CAD build for the part. Positions are in the model's coordinates, mm. Face numbers are marked on the shaded views. A direction names the side the tool comes from. Coordinates: 2 decimals unless noted, no trailing zeros. Loops run counter-clockwise (first coordinate to the right, second up) from the corner with the lowest first, then second, coordinate; pieces in that order, holes last. Notation, with made-up numbers: (-26, 24) - (20, 24) arc R13 cw to (20, 40) - close; hole circle Ø4 at (70.5, -7.5). An arc over 180 degrees is marked (long way). Put each result on its own line as item: value.
Autodesk Inventor part; units mm, degrees
ref_plane "YZ Plane" through (0, 0, 0) normal (1, 0, 0) x (0, 1, 0)
ref_plane "XZ Plane" through (0, 0, 0) normal (0, 1, 0) x (-1, 0, 0)
ref_plane "XY Plane" through (0, 0, 0) normal (0, 0, 1) x (1, 0, 0)
sketch "Sketch1" plane through (0, 0, 0) normal (0, 0, 1) x (1, 0, 0)
  line L0 (-490, 52) -> (490, 52)
  line L1 (490, 52) -> (490, 0)
  line L2 (490, 0) -> (-490, 0)
  line L3 (-490, 0) -> (-490, 52)
  point P0 (0, 0)
  point P1 (0, 0)
  dimension "d0" = 980
  dimension "d1" = 52
extrude "Plate1" add sketch "Sketch1" along normal blind 2
sketch "Sketch2" plane through (490, 2, 0) normal (0, -1, 0) x (1, 0, 0)
  line L0 (-980, 0) -> (0, 0)
  line L1 (0, 0) -> (0, 20)
  line L2 (0, 20) -> (-980, 20)
  line L3 (-980, 20) -> (-980, 0)
edge flange "Flange1" height 20 angle 90 thickness 2 bend radius 2.75 thickness toward (0, -1, 0) relief round relief width 2 relief depth 1 edges at (0, 0, 2) wall of the first edge with corners at (-490, 2, 0) (490, 2, 0) (490, 2, 20) (-490, 2, 20)
bend "Bend1"
corner "Corner1"
sketch "Sketch11" plane through (0, 0, 0) normal (0, 0, 1) x (1, 0, 0)
  line L0 (-490, 52) -> (490, 52)
  circle A0 centre (0, 52) radius 30
  line L1 (-490, 0) -> (490, 0)
  line L2 (246.05, 0) -> (243.95, 0)
  line L3 (243.95, 0) -> (243.95, 27)
  line L4 (243.95, 27) -> (246.05, 27)
  line L5 (246.05, 27) -> (246.05, 0)
  line L6 (-243.95, 0) -> (-246.05, 0)
  line L7 (-246.05, 0) -> (-246.05, 27) construction
  line L8 (-246.05, 27) -> (-243.95, 27) construction
  line L9 (-243.95, 27) -> (-243.95, 0) construction
  line L10 (0, 52) -> (0, 0)
  line L11 (246.05, 27) -> (246.05, 52)
  line L12 (243.95, 27) -> (243.95, 52)
  line L13 (-243.95, 27) -> (-243.95, 52) construction
  line L14 (-246.05, 27) -> (-246.05, 52) construction
  line L15 (-490, 0) -> (-490, 52)
  circle A1 centre (490, 52) radius 30
  line L16 (490, 52) -> (490, 0)
  point P0 (30, 52)
  point P1 (-30, 52)
  point P2 (-245, 27)
  point P3 (245, 27)
  point P4 (490, 22)
  point P5 (460, 52)
  point P6 (0, 22)
  dimension "d44" = 60
  dimension "d47" = 2.1
  dimension "d49" = 490
  dimension "d50" = 27
extrude "Extrusion4" cut sketch "Sketch11" along normal through all both and the other way through all contours L10 A0 L0 | A0 L10 L1 L15 L0 | L0 L11 L4 L12 picked at (-19.7493, 49.7748)
sketch "Sketch9" plane through (0, 0, 2) normal (0, 0, 1) x (1, 0, 0)
  line L0 (456.3279, 23.6801) -> (456.3279, 11.6801) construction
  line L1 (456.3279, 11.6801) -> (256.3279, 11.6801) construction
  line L2 (256.3279, 11.6801) -> (256.3279, 23.6801) construction
  line L3 (256.3279, 23.6801) -> (456.3279, 23.6801) construction
  line L4 (-490, 52) -> (490, 52)
  point P0 (0, 0)
  point P1 (1, 52)
  dimension "d38" = 200
  dimension "d39" = 12
mark "Mark3"
equation "\"d1\" = СПИНА_Стрингер_1_высота"
equation "\"d2\" = Thickness"
equation "\"d3\" = BendReliefWidth"
equation "\"d4\" = BendReliefDepth"
equation "\"d5\" = MinimumRemnant"
equation "\"d6\" = TransitionRadius"
equation "\"d9\" = BendRadius"
equation "\"d10\" = CornerReliefSize"
equation "\"d11\" = GapSize"
equation "\"d12\" = JacobiRadiusSize"
equation "\"BendReliefWidth\" = Thickness"
equation "\"BendReliefDepth\" = 0.5 * Thickness"
equation "\"CornerReliefSize\" = 4 * Thickness"
equation "\"MinimumRemnant\" = 2 * Thickness"
equation "\"TransitionRadius\" = BendRadius"
equation "\"JacobiRadiusSize\" = BendRadius"
equation "\"GapSize\" = Thickness"
properties part number "MSC 204 STRINGER BACK ^" material "Stainless Steel"
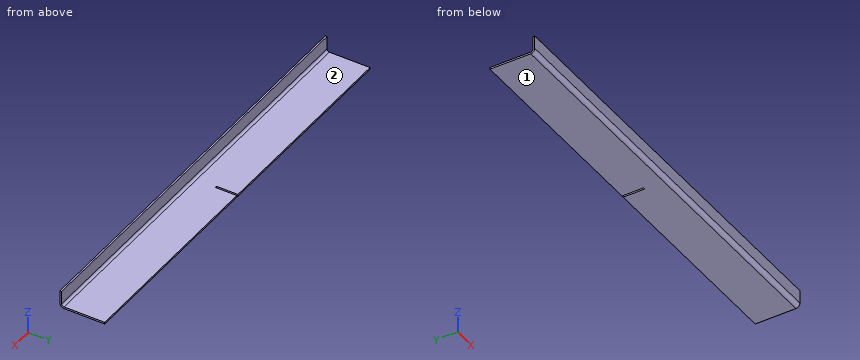
Q1. Slice it at A-A, the plane x = 141. Give the cut face in (y, z).
Determined:
outline: (0, 4.75) arc R4.75 ccw to (4.75, 0) - (52, 0) - (52, 2) - (4.75, 2) arc R2.75 cw to (2, 4.75) - (2, 20) - (0, 20) - close
Q2. Slice it at C-C, the plane z = 15. Give the cut face in (x, y).
Determined:
outline: (0, 0) - (490, 0) - (490, 2) - (0, 2) - close
Q3. Tool access for the marked faces 1 and 2: list every direction of +Z, -Z, +X, -X, +Y, -Y with a clear straight run to the whole face (end or side of a thin tool).
Determined:
face 1: -Z, +X, -X, +Y, -Y
face 2: +Z, +X, -X, +Y
Q4. Wall check: L1, parallel to Y at x = 391.5, z = 13.5; L2, parallel to Y at x = 430.5, z = 3. Give the ranges that are in metal, low to high. Write a range as from..to.
Determined:
L1: 0..2
L2: 0.33..2.63
Q5. Pin check, flat tip, straight feed: pin 1 Ø7.5 at (x, z) = (224, 11.5) entering from +Y. Stop position of the tip, or through.
Determined:
pin 1: y = 2
Q6. Slice it at B-B, the plane y = 34. Give the cut face in (x, z).
Determined:
outline: (0, 0) - (243.95, 0) - (243.95, 2) - (0, 2) - close; (246.05, 0) - (490, 0) - (490, 2) - (246.05, 2) - close
